Check sheet for the drawn part. Datum: minimum x, y, z corner. Units: mm. A direction names the side the tool comes from. Coordinates: 2 decimals unless noted, no trailing zeros. Write each loop counter-clockwise with the first axis right and the second up, starting at its lowest first coordinate (ties: lowest second). Pieces come first, ordered by that corner, then holes. Notation, with made-up numbers: M 87,-18 L 119,-18 A20 cw 119,20 Z; hole C -1.5,29 d1. An arc over 180 degrees is marked long. Answer as CSV lines item,"result".
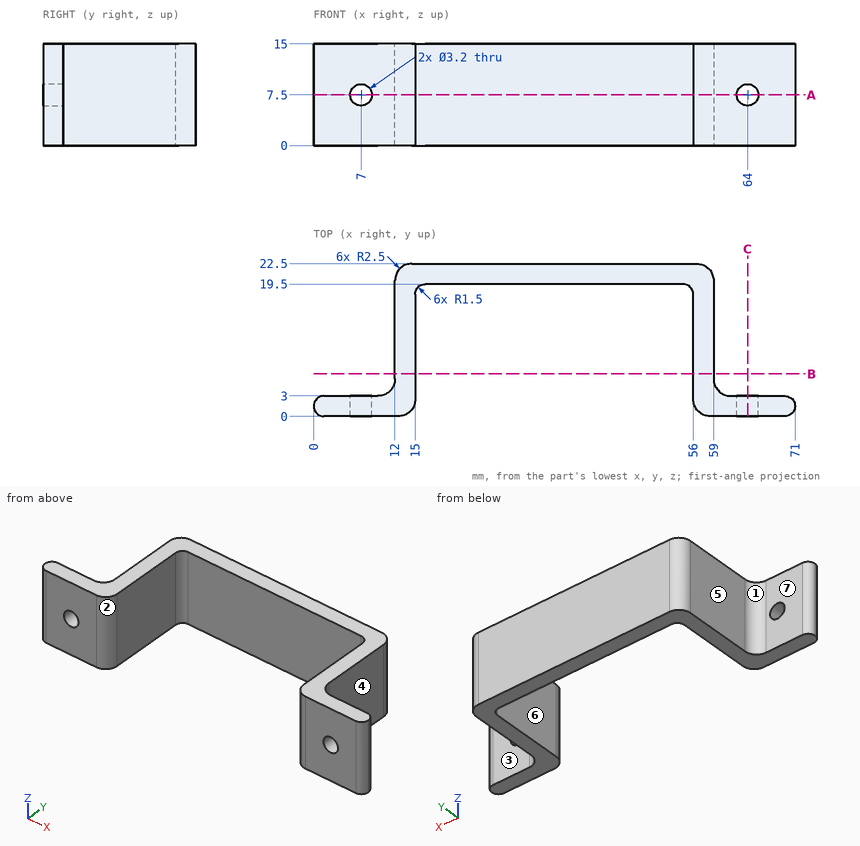
1) Tool access check on the marked faces 1, 2 and 3. Record the directions out of +Z, -Z, +X, -X, +Y, -Y that give a thin tool (end or side, any length) a straight path to the whole face; none if there is none.
Answer key:
face 1,"+Z, -Z, -X, +Y"
face 2,"+Z, -Z, -Y"
face 3,"+Z, -Z, +X, +Y"
2) Section check B-B, the plane y = 6.25. Record the boundary of the cut face in (x, z), plus the area to 3 significant figures.
Answer key:
outline,"M 12,0 L 15,0 L 15,15 L 12,15 Z; M 56,0 L 59,0 L 59,15 L 56,15 Z"
area,"90.0 mm2"
3) Mould release check, pull along X, two halves, no side actions. Record for the marked faces 4, 5, 6 and 7: pulls with the +X half, pulls with the -X half, needs draft (parallel to the pull), parting line crosses it, or undercut.
Answer key:
face 4,"pulls with the +X half"
face 5,"pulls with the -X half"
face 6,"undercut"
face 7,"needs draft"
4) Thickness scan on line 1 along X through (y, z) = (11.25, 3.5); line 2 along Z through (x, y) = (64, 1.7); line 3 along X through (y, z) = (1.25, 7.5) (1 decimal). Record the ranges inside material, lowest first.
Answer key:
line 1,"x = 12 to 15, 56 to 59"
line 2,"z = 0 to 5.9, 9.1 to 15"
line 3,"x = 0 to 5.4, 8.6 to 14.7, 56.3 to 62.4, 65.6 to 71"
5) Depth check by flat-ended pin: P1, Ø4.5, axis at y = 12.5, z = 9, coming from the -X side; P2, Ø7.5, axis at x = 28.5, z = 5, coming from the -Y side; P3, Ø12, axis at x = 13, y = 13.5, coming from the -Z side; P4, Ø9, axis at x = 4, z = 7, coming from the +Y side. Enter the tip coordinate at first touch or a pass-through.
Answer key:
P1,"stops at x = 12"
P2,"stops at y = 19.5"
P3,"stops at z = 0"
P4,"stops at y = 3"
6) Section check C-C, the plane x = 64. Record the boundary of the cut face in (y, z).
Answer key:
outline,"M 0,0 L 3,0 L 3,5.9 L 0,5.9 Z; M 0,9.1 L 3,9.1 L 3,15 L 0,15 Z"
7) Section check A-A, the plane z = 7.5. Give the number of separate pieces and of enclosed holes in the cut face, plus the area to 3 significant figures.
Answer key:
separate pieces,"3"
enclosed holes,"0"
area,"307 mm2"
